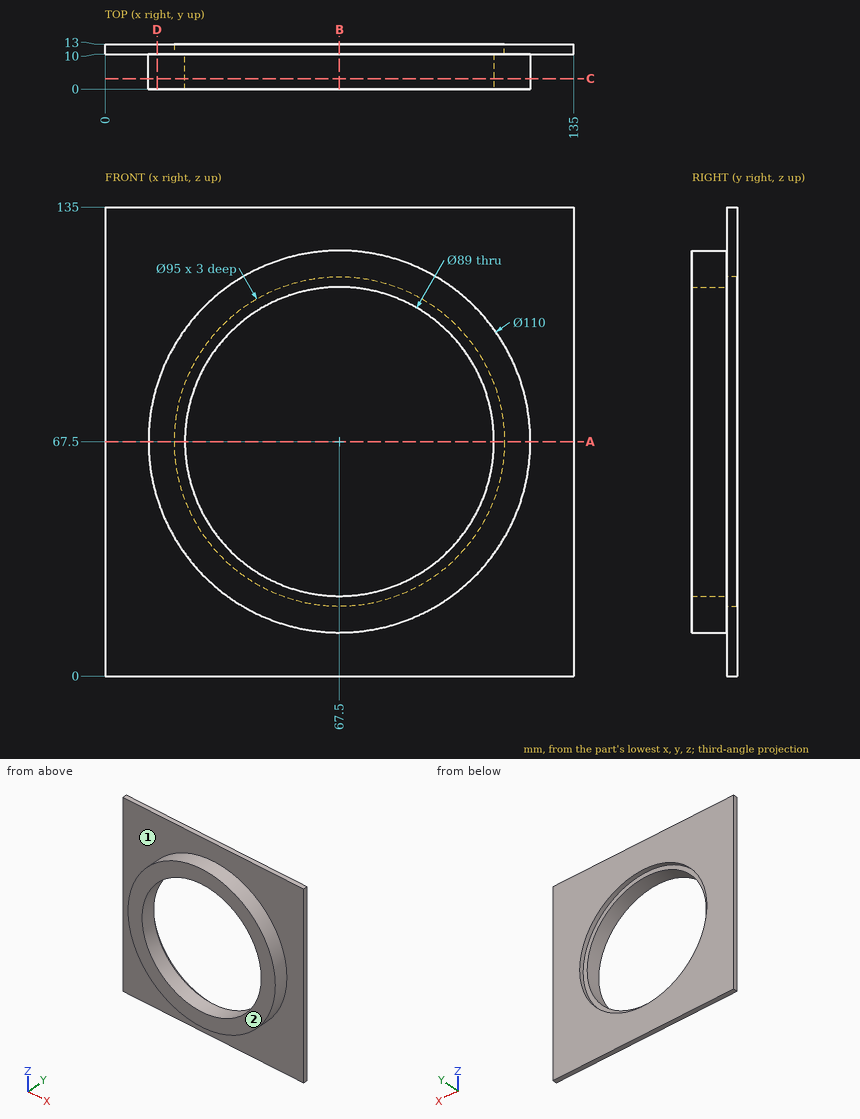
Input: dimensioned drawing with shaded views. Units: mm. Origin: part minimum x, y, z. A direction names the side the tool comes from. Give positions to 0.01 mm unless a question says otherwise; leave off trailing zeros. Order: outer loops, then holes, each group sorted by start corner. A loop starts at its lowest first (then second) coordinate and runs counter-clockwise, first axis right, second up.
(1) Section query D-D (x = 15). Return the cut outline in (y, z), plus the area to 3 significant figures.
(2) Section query C-C (y = 3). Return the cut outline in (x, z).
(3) Section query B-B (x = 67.5). Return the cut outline in (y, z), plus the area to 3 significant figures.
(4) Access query for the marked faces 1 and 2. Directions: +Z, -Z, +X, -X, +Y, -Y. A direction counts if a zero-diameter tool reaches every point of the face in a straight line with its end or side. Return the directions, or none.
(5) Section query A-A (z = 67.5). Return the cut outline in (x, y).
(6) Material intervals for line 1 along Z through (x, y) = (67.5, 11.15); line 2 along Y through (x, z) = (21, 109); line 3 along X through (y, z) = (6, 50.5), sorted ascending.
(7) Contact query for flat-ended pins moving along their axis: P1, Ø3, axis at y = 7.5, z = 111.5, coming from the -X side; P2, Ø1.5, axis at y = 8.5, z = 79, coming from the -X side; P3, Ø1, axis at x = 101, z = 41, coming from the -Y side. Output: stop coordinate, or through.
Outcome:
1. outline: (0, 51.11) - (10, 51.11) - (10, 0) - (13, 0) - (13, 135) - (10, 135) - (10, 83.89) - (0, 83.89) - close
1. area: 733 mm2
2. outline: circle Ø110 at (67.5, 67.5); hole circle Ø89 at (67.5, 67.5)
3. outline: (0, 12.5) - (10, 12.5) - (10, 0) - (13, 0) - (13, 20) - (10, 20) - (10, 23) - (0, 23) - close; (0, 112) - (10, 112) - (10, 115) - (13, 115) - (13, 135) - (10, 135) - (10, 122.5) - (0, 122.5) - close
3. area: 330 mm2
4. face 1: -Y
4. face 2: +Z, -Z, +X, -X, -Y
5. outline: (0, 10) - (12.5, 10) - (12.5, 0) - (23, 0) - (23, 10) - (20, 10) - (20, 13) - (0, 13) - close; (112, 0) - (122.5, 0) - (122.5, 10) - (135, 10) - (135, 13) - (115, 13) - (115, 10) - (112, 10) - close
6. line 1: z = 0 to 20, 115 to 135
6. line 2: y = 10 to 13
6. line 3: x = 15.19 to 26.38, 108.62 to 119.81
7. P1: stops at x = 32.59
7. P2: stops at x = 13.56
7. P3: passes through
